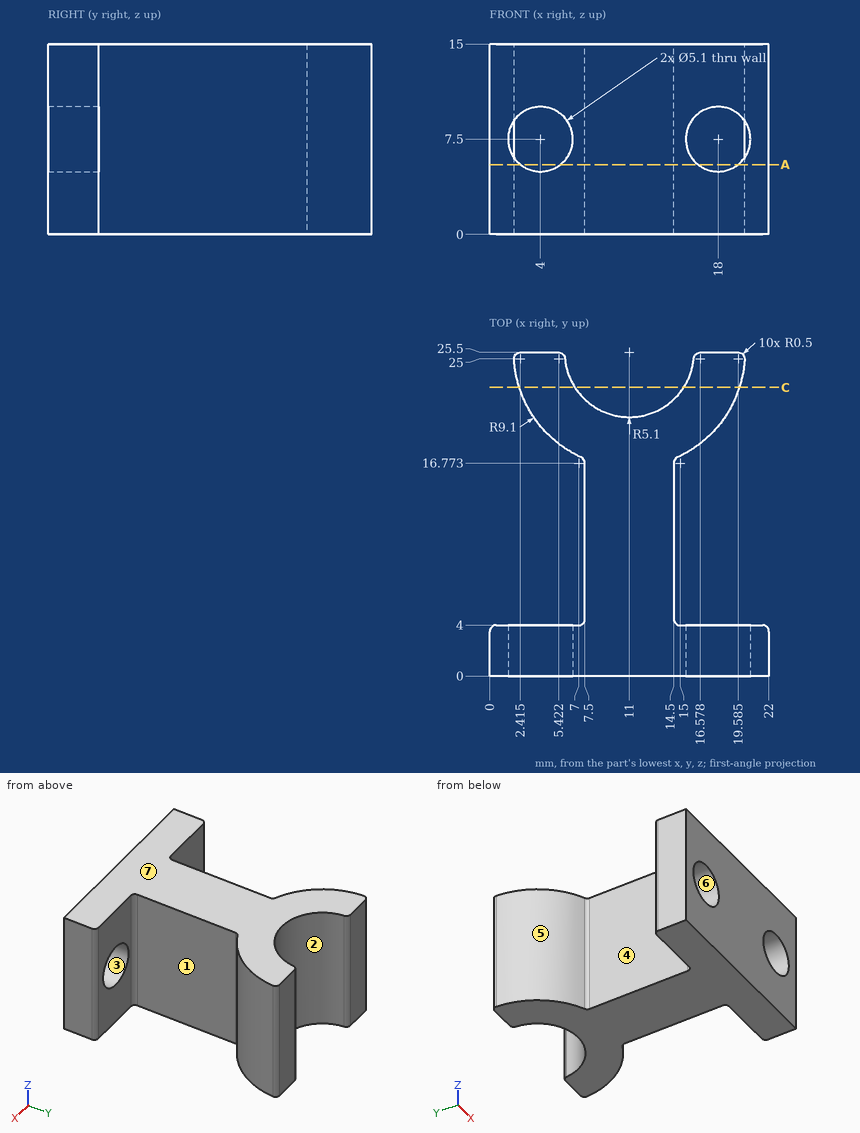
Input: dimensioned drawing with shaded views. Units: mm. Origin: part minimum x, y, z. A direction names the side the tool comes from. Give positions to 0.01 mm unless a question says otherwise; leave off trailing zeros. Loops run counter-clockwise (first coordinate to the right, second up) from the corner with the lowest first, then second, coordinate; pieces in that order, holes last. Notation, with made-up numbers: M 76.25,88.25 L 89.25,88.25 A27 cw 89.25,120.25 Z; hole C 5.25,-24.75 d5. An arc over 180 degrees is marked long. Put each result on its own line as item: value. Start each with the question number.
1) Access query for the marked faces 1, 2, 3 and 4. Directions: +Z, -Z, +X, -X, +Y, -Y. A direction counts if a zero-diameter tool reaches every point of the face in a straight line with its end or side. Return the directions, or none.
2) Cut plane C-C (y = 22.75). Output: boundary loops of the cut face in (x, z) (1 decimal).
3) Ray query, line 1 along Z through (x, y) = (18, 2.45); line 2 along X through (y, z) = (1.25, 8.5) (1 decimal); line 3 along X through (y, z) = (23.25, 10.25). Return the intervals inside material, ascending.
4) Contact query for flat-ended pins moving along their axis: pin 1 (1.5 mm diameter, centred on y = 18, z = 5, fed in from -X) (1 decimal); pin 2 (6 mm diameter, centred on y = 8.5, z = 9, fed in from +X); pin 3 (2 mm diameter, centred on y = 17, z = 13.5, fed in from -X) (1 decimal). Output: stop coordinate, or through.
5) Cut plane A-A (z = 5.5). Give the number of separate pieces and of enclosed holes in the cut face, then the cut area to 3 significant figures.
6) Pull-direction query (Z, two-part tool) for the marked faces 5, 6 and 7; classes: pulls with the +Z half, pulls with the -Z half, needs draft (parallel to the pull), parting line crosses it, or undercut.
Verdict:
1. face 1: +Z, -Z, +X
1. face 2: +Z, -Z, +Y
1. face 3: -Y
1. face 4: +Z, -Z, -X
2. outline: M 2.3,0 L 6.7,0 L 6.7,15 L 2.3,15 Z; M 15.3,0 L 19.7,0 L 19.7,15 L 15.3,15 Z
3. line 1: 0 to 4.95, 10.05 to 15
3. line 2: 0 to 1.7, 6.3 to 15.7, 20.3 to 22
3. line 3: 2.18 to 6.42, 15.58 to 19.82
4. pin 1: x = 4.9
4. pin 2: x = 14.5
4. pin 3: x = 5.8
5. separate pieces: 3
5. enclosed holes: 0
5. area: 240 mm2
6. face 5: needs draft
6. face 6: undercut
6. face 7: pulls with the +Z half
